```python
from build123d import *

# Parameters (mm, degrees)
SKETCH_1_W          = 100
SKETCH_1_H          = 20
EXTRUDE_1_DEPTH     = 7.3
SKETCH_2_R          = 2.1
CUT_EXTRUDE_1_DEPTH = 103.241332151
FILLET_1_R          = 5


with BuildPart() as part:
    # 草图1 → 凸台-拉伸1 (new body)
    with BuildSketch(Plane.XY):
        with Locations((50, 10)):
            Rectangle(SKETCH_1_W, SKETCH_1_H)
    extrude(amount=EXTRUDE_1_DEPTH)

    # 草图2 → 切除-拉伸1 (cut, through all)
    with BuildSketch(Plane.XY.offset(7.3)):
        with Locations((10, 10)):
            Circle(SKETCH_2_R)
        with Locations((50, 10)):
            Circle(SKETCH_2_R)
        with Locations((90, 10)):
            Circle(SKETCH_2_R)
    extrude(amount=-CUT_EXTRUDE_1_DEPTH, mode=Mode.SUBTRACT)

    # 圆角1
    fillet_1_edges = [part.edges().sort_by_distance(p)[0] for p in [
        (0, 20, 3.65),
        (100, 20, 3.65),
        (100, 0, 3.65),
        (0, 0, 3.65),
    ]]
    fillet(fillet_1_edges, radius=FILLET_1_R)


solid = part.part
```
Build history of the part. All positions in model axes, mm. Give positions to 0.01 mm unless a question says otherwise; leave off trailing zeros. Order: outer loops, then holes, each group sorted by start corner. A loop starts at its lowest first (then second) coordinate and runs counter-clockwise, first axis right, second up. Notation, with made-up numbers: M 86.5,63.25 L 121.5,63.25 A30 cw 121.5,95.25 Z; hole C -9.5,50 d3. An arc over 180 degrees is marked long. Write item = value, one per line. Start each with the question number.
(1) Slice it at A-A on x = 10. Write the cut outline in (y, z), plus the area to 3 significant figures.
(2) Slice it at D-D on y = 18.75. Write the cut outline in (x, z).
(3) Slice it at C-C on z = 1. Write the cut outline in (x, y).
(4) Two-plate mould, pull along X, no slides. Class faces 1 (the cylindrical face through (1, 2, 4)), 2 (the cylindrical face through (87.9, 10.09, 3.7)), 3 (the cylindrical face through (98, 19, 4)): released by +X, released by -X, zero draft, split by the parting line, or undercut.
(5) Probe L1, parallel to X at y = 10.25, z = 0.5; L2, parallel to Y at x = 90, z = 2.75; L3, parallel to Y at x = 95.5, z = 2. List the from-to ranges inside material, lowest first. Write a range as [from, to].
(6) Slice it at B-B on y = 10. Write the cut outline in (x, z), plus the area to 3 significant figures.
Responses:
q1.outline = M 0,0 L 7.9,0 L 7.9,7.3 L 0,7.3 Z; M 12.1,0 L 20,0 L 20,7.3 L 12.1,7.3 Z
q1.area = 115 mm2
q2.outline = M 1.69,0 L 98.31,0 L 98.31,7.3 L 1.69,7.3 Z
q3.outline = M 0,5 A5 ccw 5,0 L 95,0 A5 ccw 100,5 L 100,15 A5 ccw 95,20 L 5,20 A5 ccw 0,15 Z; hole C 10,10 d4.2; hole C 50,10 d4.2; hole C 90,10 d4.2
q4.face_1 = released by -X
q4.face_2 = undercut
q4.face_3 = released by +X
q5.L1 = [0, 7.91], [12.09, 47.91], [52.09, 87.91], [92.09, 100]
q5.L2 = [0, 7.9], [12.1, 20]
q5.L3 = [0.03, 19.97]
q6.outline = M 0,0 L 7.9,0 L 7.9,7.3 L 0,7.3 Z; M 12.1,0 L 47.9,0 L 47.9,7.3 L 12.1,7.3 Z; M 52.1,0 L 87.9,0 L 87.9,7.3 L 52.1,7.3 Z; M 92.1,0 L 100,0 L 100,7.3 L 92.1,7.3 Z
q6.area = 638 mm2
